```python
from build123d import *

# Parameters (mm, degrees)
SKETCH1_W           = 22
SKETCH1_H           = 10
BOSS_EXTRUDE1_DEPTH = 28
SKETCH2_R           = 3
CUT_EXTRUDE2_DEPTH  = 5
SKETCH4_W           = 22
SKETCH4_H           = 10
CUT_EXTRUDE4_DEPTH  = 32.701734968
SKETCH5_R           = 5
CUT_EXTRUDE5_DEPTH  = 5
FILLET2_R           = 10


with BuildPart() as part:
    # Sketch1 → Boss-Extrude1 (new body)
    with BuildSketch(Plane(origin=(0, 0, 0), x_dir=(1, 0, 0), z_dir=(0, 1, 0))):
        Rectangle(SKETCH1_W, SKETCH1_H)
    extrude(amount=BOSS_EXTRUDE1_DEPTH)

    # Sketch2 → Cut-Extrude2 (cut)
    with BuildSketch(Plane(origin=(0, 28, 0), x_dir=(1, 0, 0), z_dir=(0, 1, 0))):
        with Locations(Location((-6, 0, 0), (0, 0, 270))):
            Circle(SKETCH2_R)
        with Locations(Location((6, 0, 0), (0, 0, 270))):
            Circle(SKETCH2_R)
    extrude(amount=-CUT_EXTRUDE2_DEPTH, mode=Mode.SUBTRACT)

    # Sketch4 → Cut-Extrude4 (cut, through all)
    with BuildSketch(Plane(origin=(0, 0, -5), x_dir=(-1, 0, 0), z_dir=(0, 0, -1))):
        with Locations((0, 5)):
            Rectangle(SKETCH4_W, SKETCH4_H)
    extrude(amount=-CUT_EXTRUDE4_DEPTH, mode=Mode.SUBTRACT)

    # Sketch5 → Cut-Extrude5 (cut)
    with BuildSketch(Plane(origin=(0, 0, -5), x_dir=(-1, 0, 0), z_dir=(0, 0, -1))):
        with Locations((0, 17)):
            Circle(SKETCH5_R)
    extrude(amount=-CUT_EXTRUDE5_DEPTH, mode=Mode.SUBTRACT)

    # Fillet2
    fillet2_edges = [part.edges().sort_by_distance(p)[0] for p in [
        (-11, 10, 0),
        (11, 10, 0),
    ]]
    fillet(fillet2_edges, radius=FILLET2_R)


solid = part.part
```
Model file for the job. Use its own axes, mm. A direction names the side the tool comes from. Give positions to 0.01 mm unless a question says otherwise; leave off trailing zeros. Loops run counter-clockwise (first coordinate to the right, second up) from the corner with the lowest first, then second, coordinate; pieces in that order, holes last. Notation, with made-up numbers: (18.5, 49) - (65.5, 49) arc R13 cw to (65.5, 72) - close; hole circle Ø4 at (77, 73.25). An arc over 180 degrees is marked (long way). One line per item, written item: value. Start each with the question number.
1. Pin check, flat tips, straight feed: pin 1 (2 mm diameter, centred on y = 13, z = 2, fed in from -X); pin 2 (1.5 mm diameter, centred on x = 5, z = -2, fed in from -Y); pin 3 (6 mm diameter, centred on x = 5, z = 1, fed in from -Y). Stop position of each tip, or through.
2. Pull direction Z, two halves, no side cores. Call faces 4 (the cylindrical face through (3.07, 25.54, -0.65)), 5 (the flat face through (0, 17, 0)), 6 (the flat face through (0, 19, 5)): pulls with the +Z half, pulls with the -Z half, needs draft (parallel to the pull), parting line crosses it, or undercut.
3. Slice it at C-C (y = 17). List the corners of the cut face in (x, z).
4. Probe L1, parallel to X at y = 26.6, z = 0; L2, parallel to X at y = 26.5, z = 0.75; L3, parallel to Y at x = 0, z = -3.4. List the from-to ranges inside material, lowest first. Write a range as from..to.
5. Slice it at D-D (x = -4.5). List the corners of the cut face in (y, z), plus the area to 3 significant figures.
6. Which spindle directions (+Z, -Z, +X, -X, +Y, -Y) get a long thin tool onto all of the face, cutting with end or side? Do faces 1 (the cylindrical face through (-8.15, 13.01, 0.07)), 2 (the flat face through (-6, 23, 0)), 3 (the cylindrical face through (1.08, 12.12, -2.54)). Say none if no direction does.
7. Slice it at A-A (y = 24). List the corners of the cut face in (x, z).
8. Slice it at B-B (x = 6). List the corners of the cut face in (y, z).
Solution:
1. pin 1: stops at x = -9
1. pin 2: stops at y = 10.54
1. pin 3: stops at y = 10.05
2. face 4: undercut
2. face 5: pulls with the -Z half
2. face 6: pulls with the +Z half
3. outline: (-10.54, -5) - (-5, -5) - (-5, 0) - (5, 0) - (5, -5) - (10.54, -5) - (10.54, 5) - (-10.54, 5) - close
4. L1: x = -11..-9, -3..3, 9..11
4. L2: x = -11..-8.9, -3.1..3.1, 8.9..11
4. L3: y = 10..12, 22..28
5. outline: (10.63, -5) - (14.82, -5) - (14.82, 0) - (19.18, 0) - (19.18, -5) - (28, -5) - (28, -2.6) - (23, -2.6) - (23, 2.6) - (28, 2.6) - (28, 5) - (10.63, 5) - close
5. area: 126 mm^2
6. face 1: +Z, -Z, -X, -Y
6. face 2: +Y
6. face 3: -Z
7. outline: (-11, -5) - (11, -5) - (11, 5) - (-11, 5) - close; hole circle Ø6 at (-6, 0); hole circle Ø6 at (6, 0)
8. outline: (11.34, -5) - (28, -5) - (28, -3) - (23, -3) - (23, 3) - (28, 3) - (28, 5) - (11.34, 5) - close
